Design review of the part built by this model. Coordinates are the model's own, in mm. A direction names the side the tool comes from. Coordinates: 2 decimals unless noted, no trailing zeros. Loops run counter-clockwise (first coordinate to the right, second up) from the corner with the lowest first, then second, coordinate; pieces in that order, holes last. Notation, with made-up numbers: (59, 64.25) -> (73, 64.25) arc R27 ccw to (73, 91.25) -> close; hole circle Ø2 at (38.5, 72.5). An arc over 180 degrees is marked (long way). Use a Markdown table: item, result. Add a question column.
Q1. Take a section at D-D on z = 18.5. Write out the cut boundary in (x, y).
Q2. Take a section at A-A on z = 7. Write out the cut boundary in (x, y).
Q3. Take a section at C-C on y = 0. Write out the cut boundary in (x, z), plus the area to 3 significant figures.
Q4. For faces 5 (the face through (-1.08, -4.88, 30.59)), 6 (the face through (-3, -18, 30)), 7 (the face through (-3, 17, 30)), list the 3-axis set-ups (+Z, -Z, +X, -X, +Y, -Y) from which the entire face can be reached by the end or side of a thin tool; tool diameter is ignored.
Q5. Take a section at B-B on y = -17.5. Write out the cut boundary in (x, z), plus the area to 3 significant figures.
Q6. Draft analysis for pull direction X (two halves, no side actions). For faces 1 (the face through (9, 0, 30)), 2 (the face through (0, 0, 2)), 3 (the face through (-5, 20, 7)), 4 (the face through (-7, 0, 30)), state which applies: pulls with the +X half, pulls with the -X half, needs draft (parallel to the pull), parting line crosses it, or undercut.
Q7. For probe 1 along Z at (x, y) = (-5.15, -17.5); probe 2 along Z at (x, y) = (0.5, -4); probe 3 along X at (y, z) = (18.5, 22), list the stretches that pass through material, from the lowest coordinate up.
Q8. Clearance check with flat-ended pins moving along their axes: pin 1 Ø5.5 at (y, z) = (18, 24.5) entering from +X; pin 2 Ø6 at (y, z) = (-9, 9.5) entering from +X. State where each tip first meets the part, or that it passes through.
from build123d import *

# Parameters (mm, degrees)
F0_R     = 5
F1_DEPTH = 2
F2_R     = 5
F3_DEPTH = 58
F4_R     = 2.5
F5_DEPTH = 10


with BuildPart() as f1:
    # F0 (on Top) → F1 (new body)
    with BuildSketch(Plane.XY):
        with BuildLine():
            ThreePointArc((-3, -12), (-2.12132, -9.87868), (0, -9))
            ThreePointArc((0, -9), (9, 0), (0, 9))
            ThreePointArc((0, 9), (-2.12132, 9.87868), (-3, 12))
            Line((-3, 12), (-3, 23))
            Line((-3, 23), (-7, 23))
            Line((-7, 23), (-7, -23))
            Line((-7, -23), (-3, -23))
            Line((-3, -23), (-3, -12))
        make_face()
        Circle(F0_R, mode=Mode.SUBTRACT)
        Circle(F0_R)
    extrude(amount=F1_DEPTH)

    # F2 (on face) → F3 (join)
    with BuildSketch(Plane.XY.offset(2)):
        with BuildLine():
            ThreePointArc((-3, -12), (-2.12132, -9.87868), (0, -9))
            ThreePointArc((0, -9), (9, 0), (0, 9))
            ThreePointArc((0, 9), (-2.12132, 9.87868), (-3, 12))
            Line((-3, 12), (-3, 23))
            Line((-3, 23), (-7, 23))
            Line((-7, 23), (-7, -23))
            Line((-7, -23), (-3, -23))
            Line((-3, -23), (-3, -12))
        make_face()
        with Locations((0, 0)):
            Circle(F2_R, mode=Mode.SUBTRACT)
    extrude(amount=F3_DEPTH)

    # F4 (on face) → F5 (cut)
    with BuildSketch(Plane(origin=(-7, 0, 0), x_dir=(0, -1, 0), z_dir=(-1, 0, 0))):
        with Locations((-17.5, 53)):
            Circle(F4_R)
        with Locations((17.5, 7)):
            Circle(F4_R)
        with Locations((-17.5, 7)):
            Circle(F4_R)
        with Locations((17.5, 53)):
            Circle(F4_R)
    extrude(amount=-F5_DEPTH, mode=Mode.SUBTRACT)


solid = f1.part
Answer list:
| question | item | result |
|---|---|---|
| 1 | outline | (-7, -23) -> (-3, -23) -> (-3, -12) arc R3 cw to (0, -9) arc R9 ccw to (0, 9) arc R3 cw to (-3, 12) -> (-3, 23) -> (-7, 23) -> close; hole circle Ø10 at (0, 0) |
| 2 | outline | (-7, -23) -> (-3, -23) -> (-3, -20) -> (-7, -20) -> close; (-7, -15) -> (-3, -15) -> (-3, -12) arc R3 cw to (0, -9) arc R9 ccw to (0, 9) arc R3 cw to (-3, 12) -> (-3, 15) -> (-7, 15) -> close; (-7, 20) -> (-3, 20) -> (-3, 23) -> (-7, 23) -> close; hole circle Ø10 at (0, 0) |
| 3 | outline | (-7, 0) -> (9, 0) -> (9, 60) -> (5, 60) -> (5, 2) -> (-5, 2) -> (-5, 60) -> (-7, 60) -> close |
| 3 | area | 380 mm² |
| 4 | face 5 | +Z |
| 4 | face 6 | +Z, -Z, +X, -Y |
| 4 | face 7 | +Z, -Z, +X, +Y |
| 5 | outline | (-7, 0) -> (-3, 0) -> (-3, 4.5) -> (-7, 4.5) -> close; (-7, 9.5) -> (-3, 9.5) -> (-3, 50.5) -> (-7, 50.5) -> close; (-7, 55.5) -> (-3, 55.5) -> (-3, 60) -> (-7, 60) -> close |
| 5 | area | 200 mm² |
| 6 | face 1 | pulls with the +X half |
| 6 | face 2 | undercut |
| 6 | face 3 | needs draft |
| 6 | face 4 | pulls with the -X half |
| 7 | probe 1 | 0 to 4.5, 9.5 to 50.5, 55.5 to 60 |
| 7 | probe 2 | 0 to 2 |
| 7 | probe 3 | -7 to -3 |
| 8 | pin 1 | x = -3 |
| 8 | pin 2 | x = 6.71 |
